Could you check a few things on this model? Use its own coordinates, in mm. A direction names the side the tool comes from. Give positions to 0.01 mm unless a question says otherwise; leave off trailing zeros. Write each loop counter-clockwise with the first axis right and the second up, starting at its lowest first coordinate (ties: lowest second). Pieces come first, ordered by that corner, then holes. Notation, with made-up numbers: (6.25, -8) - (45.25, -8) arc R19 ccw to (45.25, -3) - close; hole circle Ø2 at (-29.5, 8.5). An arc over 180 degrees is marked (long way). Answer as CSV lines item,"result". Start each with the question number.
Q1. Imagine slicing it at B-B on x = -1.5. State how many separate pieces and enclosed holes the cut face has, and give its area (3 significant figures).
Q2. Imagine slicing it at A-A on x = -4.25. List the corners of the cut face in (y, z) for me.
Q3. If I drill on line 1 along Y through (x, z) = (-2, 0.3); line 2 along Z through (x, y) = (-3.5, -41); line 3 along Y through (x, z) = (-3, -0.35), over which ranges is the centre line in solid material (lowest first)?
Q4. Will these pins go through, and if not, where does the flat tip stop? pin 1 Ø4.5 at (x, y) = (-3.5, -39) entering from -Z; pin 2 Ø2 at (x, y) = (-5, -14.5) entering from -Z; pin 3 Ø1.5 at (x, y) = (-2, -13.9) entering from -Z.
Q5. On a 3-axis mill with a long thin cutter (end or side, diameter ignored), from which of +Z, -Z, +X, -X, +Y, -Y can I reach the whole of each face in a straight line? I mean faces 4 (the face through (-8.1, -16.7, -0.1)), 5 (the face through (-8.15, -37.13, -0.1)), 6 (the face through (-7.9, -41.43, 0.75)). Say none if no direction works.
Q6. We'd pull the mould along X, two halves only. Please class faces 1 (the face through (-1.423, -12.791, 0.493)), 2 (the face through (-5, -40, 0)), 3 (the face through (-7.93, -12.5, 0.75)): pulls with the +X half, pulls with the -X half, needs draft (parallel to the pull), parting line crosses it, or undercut.
Autodesk Inventor part; units mm, degrees
ref_plane "YZ Plane" through (0, 0, 0) normal (1, 0, 0) x (0, 1, 0)
ref_plane "XZ Plane" through (0, 0, 0) normal (0, 1, 0) x (-1, 0, 0)
ref_plane "XY Plane" through (0, 0, 0) normal (0, 0, 1) x (1, 0, 0)
sketch "Sketch1" plane through (0, 0, 0) normal (0, 0, 1) x (1, 0, 0)
  line L0 (-10.4863, 511.0554) -> (-10.4863, 506.5554) construction
  line L1 (-10.4863, 511.0554) -> (-10.4863, 506.5554) construction
  line L2 (-10.4863, 506.5554) -> (-10.4863, 513.0554) construction
  line L3 (-10.4863, 504.5554) -> (-10.4863, 511.0554) construction
  line L4 (-6.5, -11.9) -> (-2, -11.9)
  line L5 (0, -13.9) -> (0, -40)
  line L6 (-2, -42) -> (-6.5, -42)
  line L7 (-8.5, -40) -> (-8.5, -13.9)
  arc A0 (-6.5, -11.9) -> (-8.5, -13.9) centre (-6.5, -13.9) ccw
  arc A1 (0, -13.9) -> (-2, -11.9) centre (-2, -13.9) ccw
  arc A2 (-2, -42) -> (0, -40) centre (-2, -40) ccw
  arc A3 (-8.5, -40) -> (-6.5, -42) centre (-6.5, -40) ccw
  circle A4 centre (-2, -13.9) radius 1.25
  circle A5 centre (-2, -40) radius 1.25
  line L8 (-10.4863, 509.8054) -> (-10.4863, 512.3054)
  line L9 (-10.4863, 506.5554) -> (-10.4863, 506.5554)
  line L10 (-10.4863, 511.0554) -> (-10.4863, 513.0554)
  line L11 (-10.4863, 511.0554) -> (-10.4863, 511.0554)
  line L12 (-10.4863, 504.5554) -> (-10.4863, 506.5554)
  line L13 (-10.4863, 506.5554) -> (-10.4863, 504.5554)
  line L14 (-10.4863, 506.5554) -> (-10.4863, 506.5554)
  line L15 (-10.4863, 513.0554) -> (-10.4863, 511.0554)
  line L16 (-10.4863, 511.0554) -> (-10.4863, 511.0554)
  line L17 (-10.4863, 509.8054) -> (-10.4863, 512.3054)
  point P0 (0, 0)
  dimension "d0" = 2
extrude "Extrusion1" add sketch "Sketch1" along normal blind 1
sketch "Sketch2" plane through (0, 0, 0) normal (0, 0, -1) x (-1, 0, 0)
  line L0 (8.5, -13.9) -> (8.5, -40)
  line L1 (2, -11.9) -> (6.5, -11.9)
  line L2 (0, -40) -> (0, -13.9)
  line L3 (6.5, -42) -> (2, -42)
  line L4 (2, -15.9) -> (6.5, -15.9)
  line L5 (8.5, -17.9) -> (8.5, -36)
  line L6 (6.5, -38) -> (2, -38)
  line L7 (0, -36) -> (0, -17.9)
  arc A0 (2, -15.9) -> (0, -17.9) centre (2, -17.9) ccw
  arc A1 (8.5, -17.9) -> (6.5, -15.9) centre (6.5, -17.9) ccw
  arc A2 (6.5, -38) -> (8.5, -36) centre (6.5, -36) ccw
  arc A3 (0, -36) -> (2, -38) centre (2, -36) ccw
  point P0 (0, 0)
  point P1 (0, -15.9)
  point P2 (8.5, -38)
  dimension "d3" = 2
  dimension "d4" = 4
  dimension "d5" = 4
extrude "Extrusion2" add sketch "Sketch2" along normal blind 1
chamfer "Chamfer1" distance 0.5 angle 45 18 edges at (-0.5858, -16.4858, -1) (0, -26.95, -1) (-0.5858, -37.4142, -1) (-4.25, -38, -1) (-7.9142, -37.4142, -1) (-8.5, -26.95, -1) (-7.9142, -16.4858, -1) (-4.25, -15.9, -1) (0, -15.9, 0) (-0.5858, -12.4858, 0) (-4.25, -11.9, 0) (-7.9142, -12.4858, 0) (-8.5, -15.9, 0) (-0.5858, -41.4142, 0) (0, -38, 0) (-4.25, -42, 0) (-7.9142, -41.4142, 0) (-8.5, -38, 0)
properties part number "IO-Shield-Topplate01"
Conclusion:
1,separate pieces,"3"
1,enclosed holes,"0"
1,area,"46.8 mm^2"
2,outline,"(-42, 0.5) - (-41.5, 0) - (-38, 0) - (-38, -0.5) - (-37.5, -1) - (-16.4, -1) - (-15.9, -0.5) - (-15.9, 0) - (-12.4, 0) - (-11.9, 0.5) - (-11.9, 1) - (-42, 1) - close"
3,line 1,"-41.8 to -41.25, -38.75 to -15.15, -12.65 to -12.1"
3,line 2,"0 to 1"
3,line 3,"-38 to -15.9"
4,pin 1,"z = -1"
4,pin 2,"z = 0"
4,pin 3,"through"
5,face 4,"-Z, -X, +Y"
5,face 5,"-Z, -X, -Y"
5,face 6,"+Z, -Z, -X, -Y"
6,face 1,"undercut"
6,face 2,"needs draft"
6,face 3,"pulls with the -X half"
